For this review, take the finished solid that the model builds, in its own axes (mm). Give positions to 0.01 mm unless a question says otherwise; leave off trailing zeros. Write each loop counter-clockwise with the first axis right and the second up, starting at its lowest first coordinate (ties: lowest second). Pieces come first, ordered by that corner, then holes. Notation, with made-up numbers: M 30,-1.5 L 69,-1.5 A23 cw 69,34.5 Z; hole C -2.75,11 d3. An arc over 180 degrees is marked long. One line per item, written item: value. Start each with the question number.
Item 1: Consider section A-A, the plane x = 18.5. Write out the cut boundary in (y, z).
Item 2: Consider section C-C, the plane x = 0. Write out the cut boundary in (y, z), and give its area (3 significant figures).
Item 3: To check wall thickness, follow probe 1 along Y at (x, z) = (18.5, 1.5); probe 2 along Y at (x, z) = (0, 1.95); probe 3 along X at (y, z) = (-4, 1.4). State the ranges of each line that lie inside material, in increasing order.
Item 4: Clearance check with a flat-ended pin moving along its axis: pin 1 Ø8 at (x, y) = (-17.5, 0.5) entering from +Z. State where the tip first meets the part, or that it passes through.
Item 5: Consider section B-B, the plane z = 1.3. Write out the cut boundary in (x, y).
Autodesk Inventor part; units mm, degrees
ref_plane "YZ Plane" through (0, 0, 0) normal (1, 0, 0) x (0, 1, 0)
ref_plane "XZ Plane" through (0, 0, 0) normal (0, 1, 0) x (-1, 0, 0)
ref_plane "XY Plane" through (0, 0, 0) normal (0, 0, 1) x (1, 0, 0)
sketch "Sketch1" plane through (0, 0, 0) normal (0, 0, 1) x (1, 0, 0)
  line L0 (-45, -12.5) -> (45, -12.5)
  line L1 (45, -12.5) -> (45, 12.5)
  line L2 (45, 12.5) -> (-45, 12.5)
  line L3 (-45, 12.5) -> (-45, -12.5)
  line L4 (-45, -12.5) -> (45, 12.5) construction
  line L5 (45, -12.5) -> (-45, 12.5) construction
  circle A0 centre (-18.5, 0) radius 3.25
  circle A1 centre (18.5, 0) radius 3.25
  point P0 (0, 0)
  dimension "d0" = 90
  dimension "d1" = 25
  dimension "d2" = 37
  dimension "d3" = 18.5
  dimension "d4" = 6.5
  dimension "d5" = 6.5
  dimension "d8" = 12.5
  dimension "d9" = 12.5
extrude "Extrusion1" add sketch "Sketch1" along normal blind 3
fillet "Fillet1" radius 3 4 edges at (45, 12.5, 1.5) (45, -12.5, 1.5) (-45, 12.5, 1.5) (-45, -12.5, 1.5)
sketch "Sketch2" plane through (0, 0, 3) normal (0, 0, 1) x (1, 0, 0)
  circle A0 centre (0, 0) radius 5
  dimension "d11" = 10
extrude "Extrusion2" cut sketch "Sketch2" against normal blind 10
properties part number "de giu truc Z"
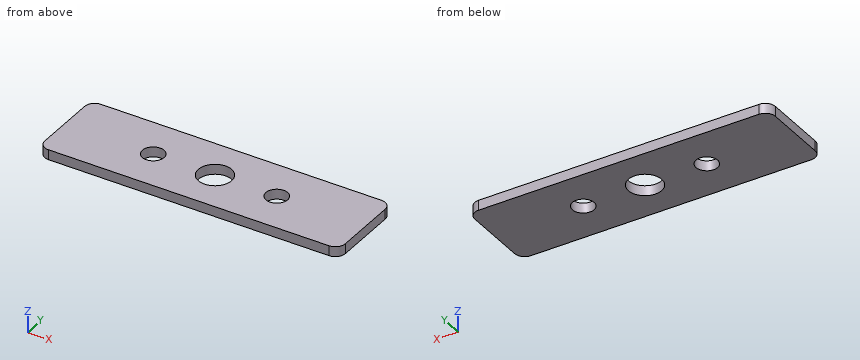
Model answer:
1. outline: M -12.5,0 L -3.25,0 L -3.25,3 L -12.5,3 Z; M 3.25,0 L 12.5,0 L 12.5,3 L 3.25,3 Z
2. outline: M -12.5,0 L -5,0 L -5,3 L -12.5,3 Z; M 5,0 L 12.5,0 L 12.5,3 L 5,3 Z
2. area: 45.0 mm2
3. probe 1: y = -12.5 to -3.25, 3.25 to 12.5
3. probe 2: y = -12.5 to -5, 5 to 12.5
3. probe 3: x = -45 to -3, 3 to 45
4. pin 1: stops at z = 3
5. outline: M -45,-9.5 A3 ccw -42,-12.5 L 42,-12.5 A3 ccw 45,-9.5 L 45,9.5 A3 ccw 42,12.5 L -42,12.5 A3 ccw -45,9.5 Z; hole C -18.5,0 d6.5; hole C 0,0 d10; hole C 18.5,0 d6.5
